```python
from build123d import *

# Parameters (mm, degrees)
F0_W     = 205
F0_H     = 420
F0_W_2   = 37.5
F0_H_2   = 355
F0_W_3   = 75
F0_H_3   = 75
F0_W_4   = 20
F0_H_4   = 85
F0_W_5   = 5
F0_H_5   = 400
F0_W_6   = 85
F0_H_6   = 35
F0_H_7   = 217.581037
F0_W_7   = 45
F0_H_8   = 312.792163
F1_DEPTH = 650
F2_W     = 10
F2_H     = 420
F3_DEPTH = 205
F4_W     = 205
F4_H     = 10
F5_DEPTH = 10


with BuildPart() as f1:
    # F0 (on Front) → F1 (new body)
    with BuildSketch(Plane.XZ):
        with Locations((-316.01329, 210)):
            Rectangle(F0_W, F0_H)
        with Locations((-374.76329, 187.5)):
            Rectangle(F0_W_2, F0_H_2, mode=Mode.SUBTRACT)
        with Locations((-327.26329, 187.5)):
            Rectangle(F0_W_2, F0_H_2, mode=Mode.SUBTRACT)
        with Locations((-261.01329, 47.5)):
            Rectangle(F0_W_3, F0_H_3, mode=Mode.SUBTRACT)
        with Locations((-288.51329, 139.707837)):
            Rectangle(F0_W_4, F0_H_4, mode=Mode.SUBTRACT)
        with Locations((-406.01329, 210)):
            Rectangle(F0_W_5, F0_H_5, mode=Mode.SUBTRACT)
        with Locations((-351.01329, 392.5)):
            Rectangle(F0_W_6, F0_H_6, mode=Mode.SUBTRACT)
        with Locations((-288.51329, 301.209481)):
            Rectangle(F0_W_4, F0_H_7, mode=Mode.SUBTRACT)
        with Locations((-246.01329, 253.603918)):
            Rectangle(F0_W_7, F0_H_8, mode=Mode.SUBTRACT)
    extrude(amount=-F1_DEPTH)

    # F2 (on face) → F3 (join, through all)
    with BuildSketch(Plane.YZ.offset(-213.51329)):
        with Locations((655, 210)):
            Rectangle(F2_W, F2_H)
    extrude(amount=-F3_DEPTH)

    # F4 (on face) → F5 (join)
    with BuildSketch(Plane.XZ):
        with Locations((-316.01329, 415)):
            Rectangle(F4_W, F4_H)
        with Locations((-316.01329, 5)):
            Rectangle(F4_W, F4_H)
    extrude(amount=F5_DEPTH)


solid = f1.part
```
For this review, take the finished solid that the model builds, in its own axes (mm). A direction names the side the tool comes from. Round coordinates to 2 decimals unless told otherwise and drop trailing zeros. Write each loop counter-clockwise with the first axis right and the second up, starting at its lowest first coordinate (ties: lowest second). Pieces come first, ordered by that corner, then holes. Notation, with made-up numbers: (79.5, 10) - (106.5, 10) arc R37 ccw to (106.5, 46) - close; hole circle Ø5 at (-36, 63.5). An arc over 180 degrees is marked (long way). Use CSV: the item, a comma, the result in double quotes.
1) The part is to be moulded in two halves that separate along X. For faces 3 (the flat face through (-213.513, 330, 207)), 4 (the flat face through (-288, 650, 300)), 5 (the flat face through (-302, 0, 226)), say which applies: pulls with the +X half, pulls with the -X half, needs draft (parallel to the pull), parting line crosses it, or undercut.
Conclusion:
face 3,"pulls with the +X half"
face 4,"undercut"
face 5,"needs draft"
2) For faces 1 (the flat face through (-246, 320, 410)), 2 (the flat face through (-418.513, 330, 207)), list the 3-axis set-ups (+Z, -Z, +X, -X, +Y, -Y) from which the entire face can be reached by the end or side of a thin tool; tool diameter is ignored.
Conclusion:
face 1,"-Y"
face 2,"+Z, -Z, -X, +Y, -Y"
3) Add section D-D on x = -246.5. Write out the cut boundary in (y, z), and give its area (3 significant figures).
Conclusion:
outline,"(-10, 0) - (660, 0) - (660, 420) - (-10, 420) - (-10, 410) - (650, 410) - (650, 97.21) - (0, 97.21) - (0, 85) - (650, 85) - (650, 10) - (-10, 10) - close"
area,"25,300 mm^2"
4) Add section B-B on z = 42.5. Write out the cut boundary in (x, y), and give its area (4 significant figures).
Conclusion:
outline,"(-418.51, 0) - (-408.51, 0) - (-408.51, 650) - (-403.51, 650) - (-403.51, 0) - (-393.51, 0) - (-393.51, 650) - (-356.01, 650) - (-356.01, 0) - (-346.01, 0) - (-346.01, 650) - (-308.51, 650) - (-308.51, 0) - (-298.51, 0) - (-298.51, 650) - (-223.51, 650) - (-223.51, 0) - (-213.51, 0) - (-213.51, 660) - (-418.51, 660) - close"
area,"34,550 mm^2"
5) Clearance check with flat-ended pins moving along their axes: pin 1 Ø10 at (x, z) = (-288, 258.5) entering from -Y; pin 2 Ø10 at (x, z) = (-342, 347.5) entering from -Y. State where each tip first meets the part, or that it passes through.
Conclusion:
pin 1,"stops at y = 650"
pin 2,"stops at y = 0"
6) Wall thickness on line 1 along Z through (x, y) = (-247, 188); line 2 along Z through (x, y) = (-387.5, 272.5); line 3 along X through (y, z) = (165, 145): over which ranges is each line inside the solid? List them lowest first. Write a range as from..to.
Conclusion:
line 1,"z = 0..10, 85..97.21, 410..420"
line 2,"z = 0..10, 365..375, 410..420"
line 3,"x = -418.51..-408.51, -403.51..-393.51, -356.01..-346.01, -308.51..-298.51, -278.51..-268.51, -223.51..-213.51"
7) Add section C-C on y = 312. Count the separate pieces of the cut face and the enclosed holes in it, and give its area (3 significant figures).
Conclusion:
separate pieces,"1"
enclosed holes,"8"
area,"28,700 mm^2"
8) Add section A-A on x = -325. Write out the cut boundary in (y, z), and give its area (3 significant figures).
Conclusion:
outline,"(-10, 0) - (660, 0) - (660, 420) - (-10, 420) - (-10, 410) - (650, 410) - (650, 375) - (0, 375) - (0, 365) - (650, 365) - (650, 10) - (-10, 10) - close"
area,"23,900 mm^2"
